```python
from build123d import *

# Parameters (mm, degrees)
SKETCH1_W           = 42
SKETCH1_H           = 42
BOSS_EXTRUDE1_DEPTH = 24
SKETCH2_W           = 16
SKETCH2_H           = 9
BOSS_EXTRUDE2_DEPTH = 5
SKETCH3_R           = 11
SKETCH3_R_2         = 4.5
BOSS_EXTRUDE4_DEPTH = 2
BOSS_EXTRUDE5_DEPTH = 22
CHAMFER1_SIZE       = 4
CHAMFER2_SIZE       = 4
CHAMFER3_SIZE       = 4
CHAMFER4_SIZE       = 4


with BuildPart() as part:
    # Sketch1 → Boss-Extrude1 (new body)
    with BuildSketch(Plane(origin=(0, 0, 0), x_dir=(1, 0, 0), z_dir=(0, 1, 0))):
        with Locations((21, 21)):
            Rectangle(SKETCH1_W, SKETCH1_H)
    extrude(amount=BOSS_EXTRUDE1_DEPTH)

    # Sketch2 → Boss-Extrude2 (add)
    with BuildSketch(Plane.XY):
        with Locations((21, 4.5)):
            Rectangle(SKETCH2_W, SKETCH2_H)
    extrude(amount=BOSS_EXTRUDE2_DEPTH)

    # Sketch3 → Boss-Extrude4 (add)
    with BuildSketch(Plane(origin=(0, 24, 0), x_dir=(1, 0, 0), z_dir=(0, 1, 0))):
        with Locations((21, 21)):
            Circle(SKETCH3_R)
        with Locations((21, 21)):
            Circle(SKETCH3_R_2, mode=Mode.SUBTRACT)
    extrude(amount=BOSS_EXTRUDE4_DEPTH)

    # Sketch4 → Boss-Extrude5 (add)
    with BuildSketch(Plane(origin=(0, 24, 0), x_dir=(1, 0, 0), z_dir=(0, 1, 0))):
        with BuildLine():
            Line((19.5, 19), (22.5, 19))
            ThreePointArc((22.5, 19), (21, 23.5), (19.5, 19))
        make_face()
    extrude(amount=BOSS_EXTRUDE5_DEPTH)

    # Chamfer1
    chamfer1_edges = [part.edges().sort_by_distance(p)[0] for p in [
        (0, 12, 0),
    ]]
    chamfer(chamfer1_edges, length=CHAMFER1_SIZE)

    # Chamfer2
    chamfer2_edges = [part.edges().sort_by_distance(p)[0] for p in [
        (42, 12, 0),
    ]]
    chamfer(chamfer2_edges, length=CHAMFER2_SIZE)

    # Chamfer3
    chamfer3_edges = [part.edges().sort_by_distance(p)[0] for p in [
        (42, 12, -42),
    ]]
    chamfer(chamfer3_edges, length=CHAMFER3_SIZE)

    # Chamfer4
    chamfer4_edges = [part.edges().sort_by_distance(p)[0] for p in [
        (0, 12, -42),
    ]]
    chamfer(chamfer4_edges, length=CHAMFER4_SIZE)


solid = part.part
```
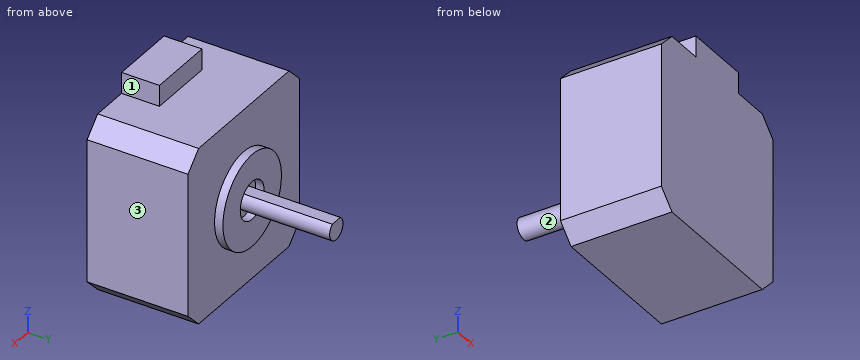
Geometry: final body of the model. Coordinates: model frame, mm. Face numbers are marked on the shaded views. A direction names the side the tool comes from. Round coordinates to 2 decimals unless told otherwise and drop trailing zeros. Write each loop counter-clockwise with the first axis right and the second up, starting at its lowest first coordinate (ties: lowest second). Pieces come first, ordered by that corner, then holes. Notation, with made-up numbers: (76.5, -31) -> (129.5, -31) arc R27 cw to (129.5, 5) -> close; hole circle Ø4 at (74, 66.25). An arc over 180 degrees is marked (long way). Use CSV: the item, a comma, the result in double quotes. Start each with the question number.
Q1. Reachability of the marked faces 1, 2 and 3 from +Z, -Z, +X, -X, +Y, -Y: full face, straight path, thin tool, end or side. Return the list, or none.
Q2. First-contact query: pin 1 Ø5 at (x, z) = (33, -24.5) entering from +Y; pin 2 Ø1.5 at (x, z) = (13, -35) entering from +Y; pin 3 Ø2 at (x, z) = (36.5, -21) entering from -Y; pin 4 Ø2.5 at (y, z) = (6, 3.5) entering from +X. Flat tips, straight axial feed; report the tip coordinate or a pass-through.
Q3. Line query: L1, parallel to X at y = 24.75, z = -21; L2, parallel to Z at x = 21, y = 25; L3, parallel to Y at x = 24, z = -21. Output: solid intervals per line, ascending.
Q4. Section C-C (x = 21). Return loops of the section in (y, z).
Q5. Section D-D (x = 14). Return loops of the section in (y, z).
Q6. Section A-A (z = -21). Return loops of the section in (x, y).
Q7. Section B-B (y = 16). Return loops of the section in (x, z), plus the area to 3 significant figures.
Result sheet:
1,face 1,"+Z, +X, +Y, -Y"
1,face 2,"+Y"
1,face 3,"+Z, -Z, +X, +Y, -Y"
2,pin 1,"y = 26"
2,pin 2,"y = 24"
2,pin 3,"y = 0"
2,pin 4,"x = 29"
3,L1,"10 to 16.5, 18.5 to 23.5, 25.5 to 32"
3,L2,"-32 to -25.5, -23.5 to -19, -16.5 to -10"
3,L3,"0 to 24"
4,outline,"(0, -42) -> (24, -42) -> (24, -32) -> (26, -32) -> (26, -25.5) -> (24, -25.5) -> (24, -23.5) -> (46, -23.5) -> (46, -19) -> (24, -19) -> (24, -16.5) -> (26, -16.5) -> (26, -10) -> (24, -10) -> (24, 0) -> (9, 0) -> (9, 5) -> (0, 5) -> close"
5,outline,"(0, -42) -> (24, -42) -> (24, -29.49) -> (26, -29.49) -> (26, -12.51) -> (24, -12.51) -> (24, 0) -> (9, 0) -> (9, 5) -> (0, 5) -> close"
6,outline,"(0, 0) -> (42, 0) -> (42, 24) -> (32, 24) -> (32, 26) -> (25.5, 26) -> (25.5, 24) -> (23.5, 24) -> (23.5, 46) -> (18.5, 46) -> (18.5, 24) -> (16.5, 24) -> (16.5, 26) -> (10, 26) -> (10, 24) -> (0, 24) -> close"
7,outline,"(0, -38) -> (4, -42) -> (38, -42) -> (42, -38) -> (42, -4) -> (38, 0) -> (4, 0) -> (0, -4) -> close"
7,area,"1,730 mm²"
